Check sheet for the modelled part. Datum: model origin and axes. Units: mm. A direction names the side the tool comes from. Round coordinates to 2 decimals unless told otherwise and drop trailing zeros. Loops run counter-clockwise (first coordinate to the right, second up) from the corner with the lowest first, then second, coordinate; pieces in that order, holes last. Notation, with made-up numbers: (14, 82.5) - (73, 82.5) arc R18 ccw to (73, 115.5) - close; hole circle Ø8 at (85, 81). An arc over 180 degrees is marked (long way). Answer in a Markdown table with one row per item. Add a question column.
(1) Cross-section at C-C on y = 60. Enter the section's corners in (x, z), then the cut area to 3 significant figures.
(2) Cross-section at B-B on z = 4.5. Enter the section's corners in (x, y), then the cut area to 3 significant figures.
(3) Cross-section at A-A on x = 19. Enter the section's corners in (y, z).
(4) Thickness scan on line 1 along Y through (x, z) = (-4, 7); line 2 along X through (y, z) = (29, 3); line 3 along X through (y, z) = (34, 6.25). Record the ranges inside material, lowest first.
(5) Access from +Z, -Z, +X, -X, +Y, -Y to the whole of each face (thin tool, end or side, straight path). Record for faces 4 (the flat face through (7, 14.539, 5)), 5 (the flat face through (-1.747, 57, 5)), 6 (the flat face through (41, 14.539, 5)).
(6) Cross-section at D-D on x = 40.5. Enter the section's corners in (y, z).
(7) Gauge pin test, flat ends, axial feed: pin 1 (4 mm diameter, centred on y = 53, z = 3.5, fed in from +X); pin 2 (0.9 mm diameter, centred on x = -3.5, z = 6.5, fed in from -Y); pin 3 (6 mm diameter, centred on x = 17.5, z = 7.5, fed in from +Y). Record the tip position at first contact, or that the pin passes through.
(8) Mould release check, pull along Y, two halves, no side actions. Record for faces 1 (the cylindrical face through (15.26, 28.32, 4.93)), 2 (the flat face through (13.253, 13, 5)), 3 (the flat face through (-3, 29.539, 5)): +Y half, -Y half, draft (parallel to the pull), parting line (faces both ways), or undercut.
from build123d import *

# Parameters (mm, degrees)
SKETCH1_R           = 4.25
BOSS_EXTRUDE1_DEPTH = 10
FILLET1_R           = 2


with BuildPart() as part:
    # Sketch1 → Boss-Extrude1 (new body)
    with BuildSketch(Plane.XY):
        Polygon((48.252973088, 14.539348583), (-1.747026912, 64.539348583), (-1.747026912, 49.539348583), (-6.747026912, 49.539348583), (-6.747026912, 29.539348583), (-1.747026912, 29.539348583), (-1.747026912, 14.539348583), (13.252973088, 14.539348583), (13.252973088, 9.539348583), (33.252973088, 9.539348583), (33.252973088, 14.539348583), align=None)
        with Locations((16.181905276, 32.468280771)):
            Circle(SKETCH1_R, mode=Mode.SUBTRACT)
    extrude(amount=BOSS_EXTRUDE1_DEPTH)

    # Fillet1
    fillet1_edges = [part.edges().sort_by_distance(p)[0] for p in [
        (-1.747026912, 14.539348583, 5),
        (13.252973088, 9.539348583, 5),
        (33.252973088, 9.539348583, 5),
        (-6.747026912, 49.539348583, 5),
        (-6.747026912, 29.539348583, 5),
    ]]
    fillet(fillet1_edges, radius=FILLET1_R)


solid = part.part
Answers:
| question | item | result |
|---|---|---|
| 1 | outline | (-1.75, 0) - (2.79, 0) - (2.79, 10) - (-1.75, 10) - close |
| 1 | area | 45.4 mm^2 |
| 2 | outline | (-6.75, 31.54) arc R2 ccw to (-4.75, 29.54) - (-1.75, 29.54) - (-1.75, 16.54) arc R2 ccw to (0.25, 14.54) - (13.25, 14.54) - (13.25, 11.54) arc R2 ccw to (15.25, 9.54) - (31.25, 9.54) arc R2 ccw to (33.25, 11.54) - (33.25, 14.54) - (48.25, 14.54) - (-1.75, 64.54) - (-1.75, 49.54) - (-4.75, 49.54) arc R2 ccw to (-6.75, 47.54) - close; hole circle Ø8.5 at (16.18, 32.47) |
| 2 | area | 1,390 mm^2 |
| 3 | outline | (9.54, 0) - (29.29, 0) - (29.29, 10) - (9.54, 10) - close; (35.65, 0) - (43.79, 0) - (43.79, 10) - (35.65, 10) - close |
| 4 | line 1 | y = 29.54 to 49.54 |
| 4 | line 2 | x = -1.75 to 13.73, 18.64 to 33.79 |
| 4 | line 3 | x = -6.75 to 12.22, 20.15 to 28.79 |
| 5 | face 4 | +Z, -Z, -X, -Y |
| 5 | face 5 | +Z, -Z, -X, +Y |
| 5 | face 6 | +Z, -Z, +X, -Y |
| 6 | outline | (14.54, 0) - (22.29, 0) - (22.29, 10) - (14.54, 10) - close |
| 7 | pin 1 | stops at x = 11.79 |
| 7 | pin 2 | stops at y = 29.54 |
| 7 | pin 3 | stops at y = 48.29 |
| 8 | face 1 | undercut |
| 8 | face 2 | draft |
| 8 | face 3 | -Y half |
